Model file for the job. Use its own axes, mm. A direction names the side the tool comes from. Round coordinates to 2 decimals unless told otherwise and drop trailing zeros. Loops run counter-clockwise (first coordinate to the right, second up) from the corner with the lowest first, then second, coordinate; pieces in that order, holes last. Notation, with made-up numbers: (56.25, -10) -> (100.25, -10) arc R20 ccw to (100.25, -2) -> close; hole circle Ø2 at (17.25, 9.5). An arc over 180 degrees is marked (long way). Use a Markdown table: item, result.
from build123d import *

# Parameters (mm, degrees)
SKETCH1_W           = 133.35
SKETCH1_H           = 101.6
BOSS_EXTRUDE1_DEPTH = 3.175
SKETCH2_W           = 3.175
SKETCH2_H           = 12.192
SKETCH2_W_2         = 19.05
SKETCH2_H_2         = 6.35
BOSS_EXTRUDE2_DEPTH = 3.175
SKETCH3_W           = 19.05
SKETCH3_H           = 6.35
SKETCH3_H_2         = 6.604
CUT_EXTRUDE1_DEPTH  = 91.306287849
SKETCH4_W           = 202.264069455
SKETCH4_H           = 60.449375303
CUT_EXTRUDE2_DEPTH  = 91.306287849


with BuildPart() as part:
    # Sketch1 → Boss-Extrude1 (new body)
    with BuildSketch(Plane(origin=(0, 0, 0), x_dir=(1, 0, 0), z_dir=(0, 1, 0))):
        Rectangle(SKETCH1_W, SKETCH1_H)
    extrude(amount=BOSS_EXTRUDE1_DEPTH)

    # Sketch2 → Boss-Extrude2 (add)
    with BuildSketch(Plane(origin=(0, 0, 0), x_dir=(-1, 0, 0), z_dir=(0, -1, 0))):
        with Locations((68.2625, -31.75)):
            Rectangle(SKETCH2_W, SKETCH2_H)
        with Locations((68.2625, -6.35)):
            Rectangle(SKETCH2_W, SKETCH2_H)
        with Locations((68.2625, 19.05)):
            Rectangle(SKETCH2_W, SKETCH2_H)
        with Locations((68.2625, 44.45)):
            Rectangle(SKETCH2_W, SKETCH2_H)
        with Locations((-68.2625, 44.45)):
            Rectangle(SKETCH2_W, SKETCH2_H)
        with Locations((-68.2625, 19.05)):
            Rectangle(SKETCH2_W, SKETCH2_H)
        with Locations((-68.2625, -6.35)):
            Rectangle(SKETCH2_W, SKETCH2_H)
        with Locations((-68.2625, -31.75)):
            Rectangle(SKETCH2_W, SKETCH2_H)
        with Locations((19.05, 53.975)):
            Rectangle(SKETCH2_W_2, SKETCH2_H_2)
        with Locations((57.15, 53.975)):
            Rectangle(SKETCH2_W_2, SKETCH2_H_2)
        with Locations((-19.05, 53.975)):
            Rectangle(SKETCH2_W_2, SKETCH2_H_2)
        with Locations((-57.15, 53.975)):
            Rectangle(SKETCH2_W_2, SKETCH2_H_2)
    extrude(amount=-BOSS_EXTRUDE2_DEPTH)

    # Sketch3 → Cut-Extrude1 (cut, through all)
    with BuildSketch(Plane(origin=(0, 0, 0), x_dir=(1, 0, 0), z_dir=(0, 1, 0))):
        with Locations((-57.15, 53.975)):
            Rectangle(SKETCH3_W, SKETCH3_H)
        with Locations((57.15, 53.848)):
            Rectangle(SKETCH3_W, SKETCH3_H_2)
    extrude(amount=CUT_EXTRUDE1_DEPTH, mode=Mode.SUBTRACT)

    # Sketch4 → Cut-Extrude2 (cut, through all)
    with BuildSketch(Plane(origin=(0, 0, 0), x_dir=(1, 0, 0), z_dir=(0, 1, 0))):
        with Locations((4.022296835, -30.224687652)):
            Rectangle(SKETCH4_W, SKETCH4_H)
    extrude(amount=CUT_EXTRUDE2_DEPTH, mode=Mode.SUBTRACT)


solid = part.part
Q1. Band-saw the part on A-A, the plane z = -54. Give the cut face in (x, y) (3 decimals).
Results list:
| item | result |
|---|---|
| outline | (-28.575, 0) -> (-9.525, 0) -> (-9.525, 3.175) -> (-28.575, 3.175) -> close; (9.525, 0) -> (28.575, 0) -> (28.575, 3.175) -> (9.525, 3.175) -> close |
Q2. Tool access for faces 1 (the face through (0, 2, -50.8)), 2 (the face through (66.675, 2, -6)), 3 (the face through (59, 2, -50.546)): list every direction of +Z, -Z, +X, -X, +Y, -Y with a clear straight run to the whole face (end or side of a thin tool).
Results list:
| item | result |
|---|---|
| face 1 | -Z, +Y, -Y |
| face 2 | +Z, +X, +Y, -Y |
| face 3 | -Z, +X, +Y, -Y |
Q3. Flat gauge pins, fed straight in: pin 1 (1 mm diameter, centred on y = 1.5, z = -7, fed in from -X) (3 decimals); pin 2 (1 mm diameter, centred on x = -35, y = 2.5, fed in from -Z); pin 3 (1.6 mm diameter, centred on x = -69, y = 1.5, fed in from +Z); pin 4 (3 mm diameter, centred on x = 48.5, z = -41, fed in from -Y). Where does each tip first touch, or does it go through?
Results list:
| item | result |
|---|---|
| pin 1 | stops at x = -66.675 |
| pin 2 | stops at z = -50.8 |
| pin 3 | stops at z = -12.95 |
| pin 4 | stops at y = 0 |
Q4. Band-saw the part on C-C, the plane x = -52. Give the cut face in (y, z) (3 decimals), plus the area to 3 significant figures.
Results list:
| item | result |
|---|---|
| outline | (0, -50.8) -> (3.175, -50.8) -> (3.175, 0) -> (0, 0) -> close |
| area | 161 mm² |
Q5. Band-saw the part on D-D, the plane z = -32. Give the cut face in (x, y) (3 decimals).
Results list:
| item | result |
|---|---|
| outline | (-66.675, 0) -> (66.675, 0) -> (66.675, 3.175) -> (-66.675, 3.175) -> close |
Q6. Pull direction X, two halves, no side cores. Call faces 4 (the face through (66.675, 2, -32)), 5 (the face through (-9.525, 2, -54)), 6 (the face through (38, 2, -50.8)): released by +X, released by -X, zero draft, split by the parting line, or undercut.
Results list:
| item | result |
|---|---|
| face 4 | released by +X |
| face 5 | undercut |
| face 6 | zero draft |
Q7. Drill centre lines: L1, parallel to X at y = 1.85, z = -53.5 (3 decimals); L2, parallel to X at y = 2.9, z = -26 (3 decimals); L3, parallel to Z at x = -8.5, y = 2.25. Where is each one in solid material? Low to high. Write a range as from..to.
Results list:
| item | result |
|---|---|
| L1 | x = -28.575..-9.525, 9.525..28.575 |
| L2 | x = -66.675..66.675 |
| L3 | z = -50.8..0 |
Q8. Band-saw the part on B-B, the plane y = 1.65. Give the cut face in (x, z) (3 decimals).
Results list:
| item | result |
|---|---|
| outline | (-69.85, -50.546) -> (-66.675, -50.546) -> (-66.675, -50.8) -> (-28.575, -50.8) -> (-28.575, -57.15) -> (-9.525, -57.15) -> (-9.525, -50.8) -> (9.525, -50.8) -> (9.525, -57.15) -> (28.575, -57.15) -> (28.575, -50.8) -> (47.625, -50.8) -> (47.625, -50.546) -> (69.85, -50.546) -> (69.85, -38.354) -> (66.675, -38.354) -> (66.675, -25.146) -> (69.85, -25.146) -> (69.85, -12.954) -> (66.675, -12.954) -> (66.675, 0) -> (-66.675, 0) -> (-66.675, -12.954) -> (-69.85, -12.954) -> (-69.85, -25.146) -> (-66.675, -25.146) -> (-66.675, -38.354) -> (-69.85, -38.354) -> close |
